```python
from build123d import *

# Parameters (mm, degrees)
TAP_DRILL_FOR_5_16_24_TAP1_D = 6.9088


with BuildPart() as part:
    # Sketch1 → Revolve1 (revolve)
    with BuildSketch(Plane.XY, mode=Mode.PRIVATE) as revolve1_sk:
        with BuildLine():
            Line((0, 0), (0, 6.447566244))
            ThreePointArc((0, 6.447566244), (0.072174996, 6.70634369), (0.267863065, 6.89041209))
            Line((0.267863065, 6.89041209), (6.2, 10))
            Line((6.2, 10), (7.7, 10))
            Line((7.7, 10), (10.7, 7))
            Line((10.7, 7), (24.9, 7))
            ThreePointArc((24.9, 7), (25.253553391, 6.853553391), (25.4, 6.5))
            Line((25.4, 6.5), (25.4, 0))
            Line((25.4, 0), (0, 0))
        make_face()
    revolve(revolve1_sk.sketch.rotate(Axis((-16.664675737, 0, 0), (1, 0, 0)), 90), axis=Axis((-16.664675737, 0, 0), (1, 0, 0)))

    # Tap Drill for 5/16-24 Tap1 (through all)
    with Locations(Plane.ZY):
        with Locations((0, 0)):
            Hole(TAP_DRILL_FOR_5_16_24_TAP1_D / 2)


solid = part.part
```
Read the model definition and answer for the solid it produces. Units are mm, in the model's axes. A direction names the side the tool comes from. Coordinates: 2 decimals unless noted, no trailing zeros. Order: outer loops, then holes, each group sorted by start corner. A loop starts at its lowest first (then second) coordinate and runs counter-clockwise, first axis right, second up. Notation, with made-up numbers: (-20, 20) - (21, 20) arc R29 ccw to (21, 48) - close; hole circle Ø1 at (25.25, 56). An arc over 180 degrees is marked (long way). Answer as a JSON object with one key per item and string values. Group by question number.
Item 1: Section C-C (x = 11.75) is taken. Give the vertices of the cut face in (y, z), plus the area to 3 significant figures.
Item 2: Consider probe 1 along Y at (x, z) = (17.5, 0); probe 2 along Z at (x, y) = (2, -0.25); probe 3 along Z at (x, y) = (18.5, 1). Determine where each line is inside the solid, lowest interval first. Write a range as from..to.
Item 3: Flat-ended cylindrical pins translate along their axes: P1, Ø3, axis at x = 5.5, y = -7.5, coming from the -Z side; P2, Ø12, axis at x = 22, y = -3, coming from the +Z side; P3, Ø8, axis at x = 18, z = -5.5, coming from the -Y side. Find the tip coordinate at first contact, or state that the pin passes through.
Item 4: Section D-D (x = 7) is taken. Give the vertices of the cut face in (y, z).
Item 5: A tool of negligible diameter and unlimited length cuts with its end or side. For faces 1 (the face through (7, 0, -10)), 2 (the face through (17.9, 6.21, 3.23)), from which of +Z, -Z, +X, -X, +Y, -Y can it reach the whole face along a straight path? Write none if from no direction.
Item 6: Section A-A (y = 0) is taken. Give the vertices of the cut face in (x, z), plus the area to 3 significant figures.
Item 7: The mould has two halves that part along Y. Classify faces 3 (the face through (0.639, 6.286, 3.269)), 4 (the face through (25.4, 3, 3)), 5 (the face through (12.878, 3.425, 0.45)): +Y half, -Y half, draft (parallel to the pull), parting line (faces both ways), or undercut.
Results are:
{
 "1": {"outline": "circle Ø14 at (0, 0); hole circle Ø6.91 at (0, 0)", "area": "116 mm^2"},
 "2": {"probe 1": "y = -7..-3.45, 3.45..7", "probe 2": "z = -7.79..-3.45, 3.45..7.79", "probe 3": "z = -6.93..-3.31, 3.31..6.93"},
 "3": {"P1": "stops at z = -7.87", "P2": "stops at z = 7", "P3": "stops at y = -6.84"},
 "4": {"outline": "circle Ø20 at (0, 0); hole circle Ø6.91 at (0, 0)"},
 "5": {"face 1": "+X, -X", "face 2": "+X"},
 "6": {"outline": "(0, -6.45) arc R0.5 ccw to (0.27, -6.89) - (6.2, -10) - (7.7, -10) - (10.7, -7) - (24.9, -7) arc R0.5 ccw to (25.4, -6.5) - (25.4, -3.45) - (0, -3.45) - close; (0, 3.45) - (25.4, 3.45) - (25.4, 6.5) arc R0.5 ccw to (24.9, 7) - (10.7, 7) - (7.7, 10) - (6.2, 10) - (0.27, 6.89) arc R0.5 ccw to (0, 6.45) - close", "area": "215 mm^2"},
 "7": {"face 3": "parting line", "face 4": "draft", "face 5": "undercut"}
}
